Job drawing, mm, ordinate dimensions from the low corner. One solid piece. Round coordinates to 2 decimals unless told otherwise and drop trailing zeros. Write each loop counter-clockwise with the first axis right and the second up, starting at its lowest first coordinate (ties: lowest second). Pieces come first, ordered by that corner, then holes.
1) Saw through at C-C on z = 2.95. Write the cut outline in (x, y), and give its area (3 significant figures).
2) Saw through at A-A on y = 27. Write the cut outline in (x, z), and give its area (3 significant figures).
3) Drill centre lines: L1, parallel to X at y = 29.5, z = 3.65; L2, parallel to X at y = 15, z = 3; L3, parallel to Y at x = 2.5, z = 2.8. Where is each one in solid material? Low to high.
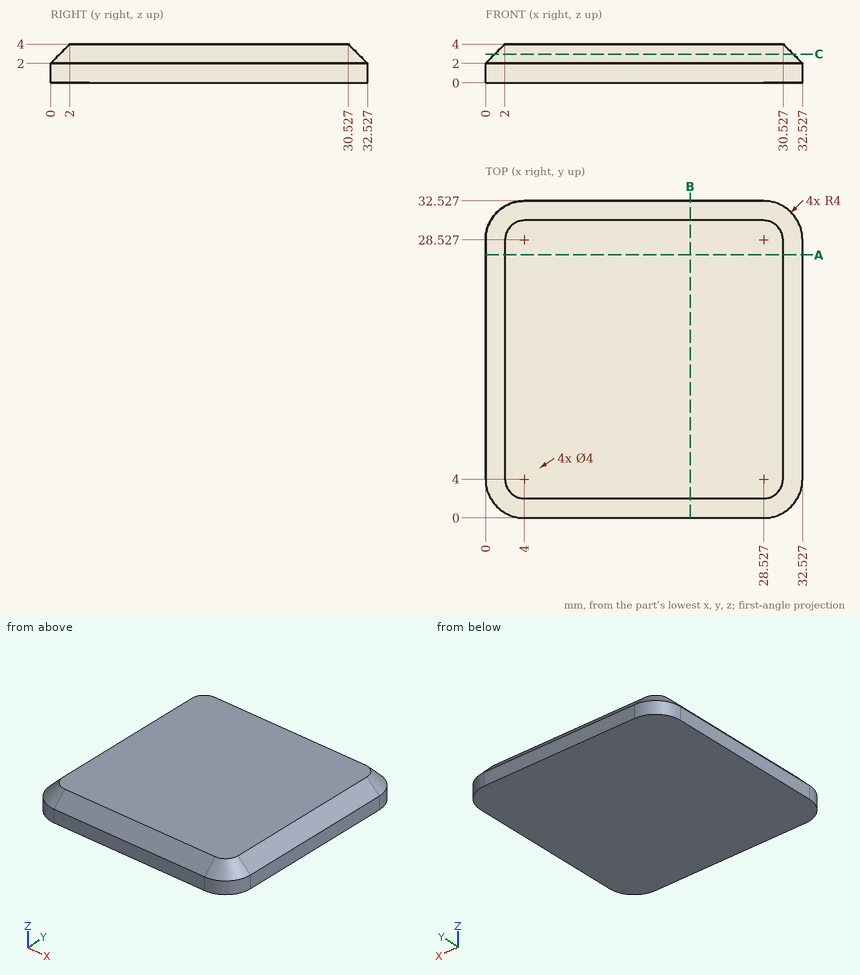
Completed:
1. outline: (0.95, 4) arc R3.05 ccw to (4, 0.95) - (28.53, 0.95) arc R3.05 ccw to (31.58, 4) - (31.58, 28.53) arc R3.05 ccw to (28.53, 31.58) - (4, 31.58) arc R3.05 ccw to (0.95, 28.53) - close
1. area: 930 mm2
2. outline: (0, 0) - (32.53, 0) - (32.53, 2) - (30.53, 4) - (2, 4) - (0, 2) - close
2. area: 126 mm2
3. L1: x = 1.86 to 30.67
3. L2: x = 1 to 31.53
3. L3: y = 1.17 to 31.35
